Build history of the part. All positions in model axes, mm. A direction names the side the tool comes from. Give positions to 0.01 mm unless a question says otherwise; leave off trailing zeros. Order: outer loops, then holes, each group sorted by start corner. A loop starts at its lowest first (then second) coordinate and runs counter-clockwise, first axis right, second up. Notation, with made-up numbers: (-16, 4.5) - (-10, 4.5) arc R25 cw to (-10, 22.5) - close; hole circle Ø9 at (15.5, 37.25). An arc over 180 degrees is marked (long way). Write each question's results on one line, items separated by ' | '. Start each with the question number.
1) Drop flat-ended pins along their axis: pin 1 Ø0.7 at (y, z) = (3.5, 0.5) entering from -X; pin 2 Ø2 at (x, z) = (1, -1.5) entering from -Y. Give the stop position or say it passes through.
2) Drill centre lines: line 1 along Y through (x, z) = (3, -1.2); line 2 along X through (y, z) = (3.25, 0); line 3 along Z through (x, y) = (-0.25, 3.7). Where is each one in solid material? Low to high. Write a range as from..to.
3) Tool access for faces 1 (the face through (-0.75, 3.3, 0)), 2 (the face through (-4, 1, 0)), 3 (the face through (0.75, 3.3, 0)): list every direction of +Z, -Z, +X, -X, +Y, -Y with a clear straight run to the whole face (end or side of a thin tool).
4) Cut at D-D on z = 0.35. List the corners of the cut face in (x, y).
5) Cut at A-A on z = 1.45. List the corners of the cut face in (x, y).
6) Cut at B-B on y = 3.4. List the corners of the cut face in (x, z).
7) Cut at C-C on x = 1.25. List the corners of the cut face in (y, z), plus the area to 3 significant figures.
from build123d import *

# Parameters (mm, degrees)
SKETCH_1_W      = 8
SKETCH_1_H      = 5
EXTRUDE_1_DEPTH = 3
EXTRUDE_2_DEPTH = 0.75
FILLET_1_R      = 1.1


with BuildPart() as part:
    # 草图1 → 凸台-拉伸1 (new body)
    with BuildSketch(Plane(origin=(0, 0, 0), x_dir=(1, 0, 0), z_dir=(0, 1, 0))):
        Rectangle(SKETCH_1_W, SKETCH_1_H)
    extrude(amount=EXTRUDE_1_DEPTH)

    # 草图2 → 凸台-拉伸2 (add, symmetric)
    with BuildSketch(Plane(origin=(0, 0, 0), x_dir=(0, 0, -1), z_dir=(1, 0, 0))):
        Polygon((0, 3.866025404), (-1.5, 3), (1.5, 3), align=None)
    extrude(amount=EXTRUDE_2_DEPTH, both=True)

    # 圆角1
    fillet_1_edges = [part.edges().sort_by_distance(p)[0] for p in [
        (0, 3, -1.5),
        (0, 3, 1.5),
    ]]
    fillet(fillet_1_edges, radius=FILLET_1_R)


solid = part.part
Results:
1) pin 1: x = -0.75 | pin 2: y = 0
2) line 1: 0..3 | line 2: -0.75..0.75 | line 3: -0.29..0.29
3) face 1: +Z, -Z, -X, +Y | face 2: +Z, -Z, -X, +Y, -Y | face 3: +Z, -Z, +X, +Y
4) outline: (-4, 0) - (4, 0) - (4, 3) - (0.75, 3) - (0.75, 3.66) - (-0.75, 3.66) - (-0.75, 3) - (-4, 3) - close
5) outline: (-4, 0) - (4, 0) - (4, 3) - (0.75, 3) - (0.75, 3.06) - (-0.75, 3.06) - (-0.75, 3) - (-4, 3) - close
6) outline: (-0.75, -0.81) - (0.75, -0.81) - (0.75, 0.81) - (-0.75, 0.81) - close
7) outline: (0, -2.5) - (3, -2.5) - (3, 2.5) - (0, 2.5) - close | area: 15.0 mm^2
